Source: CAD feature listing. Evaluate the final solid. Frame: model axes, mm. Give positions to 0.01 mm unless a question says otherwise; leave off trailing zeros. Order: outer loops, then holes, each group sorted by start corner. A loop starts at its lowest first (then second) coordinate and runs counter-clockwise, first axis right, second up. Notation, with made-up numbers: M 60.5,-39 L 87.5,-39 A23 ccw 87.5,-7 Z; hole C -6,67 d3. An arc over 180 degrees is marked long. Use CSV: the item, a comma, the result in double quotes. Start each with the question number.
1. Section query B-B, the plane x = 0. Return the cut outline in (y, z).
2. Pin query (flat end, axial travel): P1, Ø3.5, axis at x = -34.6, y = 19.98, coming from the +Z side; P2, Ø3, axis at y = -26, z = 0.5, coming from the +X side; P3, Ø1.5, axis at x = 15.5, z = 3, coming from the +Y side; P4, Ø1, axis at x = 2.5, z = 4, coming from the +Y side. Return the tip coordinate at first contact, or that it passes through.
3. Section query D-D, the plane x = 33.35. Return the cut outline in (y, z), plus the area to 3 significant figures.
4. Section query C-C, the plane z = 3.65. State how many separate pieces and enclosed holes the cut face has, plus the area to 3 significant figures.
5. Line query: line 1 along Y through (x, z) = (0, 2.35); line 2 along X through (y, z) = (-28, 3.8); line 3 along X through (y, z) = (19, 3.1). Output: solid intervals per line, ascending. Write a range as [from, to].
6. Section query A-A, the plane y = 0. Return the cut outline in (x, z), plus the area to 4 significant figures.
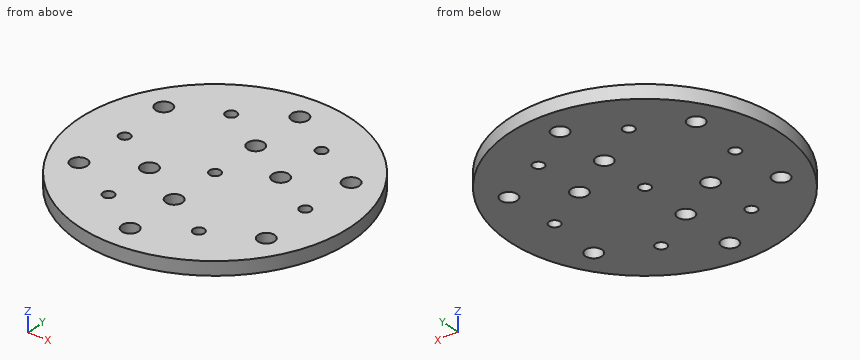
from build123d import *

# Parameters (mm, degrees)
ESQUISSE1_R        = 50
ESQUISSE1_R_2      = 3.05
ESQUISSE1_R_3      = 2.05
BOSS_EXTRU_1_DEPTH = 5


with BuildPart() as part:
    # Esquisse1 → Boss.-Extru.1 (new body)
    with BuildSketch(Plane.XY):
        Circle(ESQUISSE1_R)
        with Locations((-34.597845014, 19.975075133)):
            Circle(ESQUISSE1_R_2, mode=Mode.SUBTRACT)
        with Locations((0, 39.950150265)):
            Circle(ESQUISSE1_R_2, mode=Mode.SUBTRACT)
        with Locations((34.597845014, 19.975075133)):
            Circle(ESQUISSE1_R_2, mode=Mode.SUBTRACT)
        with Locations((34.597845014, -19.975075132)):
            Circle(ESQUISSE1_R_2, mode=Mode.SUBTRACT)
        with Locations((0, -39.950150265)):
            Circle(ESQUISSE1_R_2, mode=Mode.SUBTRACT)
        with Locations((-34.597845014, -19.975075133)):
            Circle(ESQUISSE1_R_2, mode=Mode.SUBTRACT)
        with Locations((0, 19.165334425)):
            Circle(ESQUISSE1_R_2, mode=Mode.SUBTRACT)
        with Locations((0, -19.232757636)):
            Circle(ESQUISSE1_R_2, mode=Mode.SUBTRACT)
        with Locations((-33.35, 0)):
            Circle(ESQUISSE1_R_3, mode=Mode.SUBTRACT)
        with Locations((-16.675, 28.881947216)):
            Circle(ESQUISSE1_R_3, mode=Mode.SUBTRACT)
        with Locations((16.675, 28.881947216)):
            Circle(ESQUISSE1_R_3, mode=Mode.SUBTRACT)
        with Locations((33.35, 0)):
            Circle(ESQUISSE1_R_3, mode=Mode.SUBTRACT)
        with Locations((16.675, -28.881947216)):
            Circle(ESQUISSE1_R_3, mode=Mode.SUBTRACT)
        with Locations((-16.675, -28.881947216)):
            Circle(ESQUISSE1_R_3, mode=Mode.SUBTRACT)
        Circle(ESQUISSE1_R_3, mode=Mode.SUBTRACT)
        with Locations((-16.671397033, -9.625235564)):
            Circle(ESQUISSE1_R_2, mode=Mode.SUBTRACT)
        with Locations((16.669571796, 9.624181764)):
            Circle(ESQUISSE1_R_2, mode=Mode.SUBTRACT)
    extrude(amount=BOSS_EXTRU_1_DEPTH)


solid = part.part
Result set:
1,outline,"M -50,0 L -43,0 L -43,5 L -50,5 Z; M -36.9,0 L -22.28,0 L -22.28,5 L -36.9,5 Z; M -16.18,0 L -2.05,0 L -2.05,5 L -16.18,5 Z; M 2.05,0 L 16.12,0 L 16.12,5 L 2.05,5 Z; M 22.22,0 L 36.9,0 L 36.9,5 L 22.22,5 Z; M 43,0 L 50,0 L 50,5 L 43,5 Z"
2,P1,"through"
2,P2,"x = 43.59"
2,P3,"y = 47.77"
2,P4,"y = 49.96"
3,outline,"M -37.25,0 L -22.76,0 L -22.76,5 L -37.25,5 Z; M -17.19,0 L -2.05,0 L -2.05,5 L -17.19,5 Z; M 2.05,0 L 17.19,0 L 17.19,5 L 2.05,5 Z; M 22.76,0 L 37.25,0 L 37.25,5 L 22.76,5 Z"
3,area,"296 mm2"
4,separate pieces,"1"
4,enclosed holes,"17"
4,area,"7,470 mm2"
5,line 1,"[-50, -43], [-36.9, -22.28], [-16.18, -2.05], [2.05, 16.12], [22.22, 36.9], [43, 50]"
5,line 2,"[-41.42, -18.53], [-14.82, 14.82], [18.53, 41.42]"
5,line 3,"[-46.25, -37.49], [-31.71, -3.05], [3.05, 31.71], [37.49, 46.25]"
6,outline,"M -50,0 L -35.4,0 L -35.4,5 L -50,5 Z; M -31.3,0 L -2.05,0 L -2.05,5 L -31.3,5 Z; M 2.05,0 L 31.3,0 L 31.3,5 L 2.05,5 Z; M 35.4,0 L 50,0 L 50,5 L 35.4,5 Z"
6,area,"438.5 mm2"
